Could you check a few things on this model? Use its own coordinates, in mm. Give positions to 0.01 mm unless a question says otherwise; leave off trailing zeros. Order: outer loops, then holes, each group sorted by start corner. A loop starts at its lowest first (then second) coordinate and runs counter-clockwise, first axis right, second up. Notation, with made-up numbers: M 44,-36.5 L 62,-36.5 A26 ccw 62,-11.5 Z; hole C 53.5,-20 d1. An arc over 180 degrees is marked long. Return JSON: item names as keys, results as strings. Group by question number.
```python
from build123d import *

# Parameters (mm, degrees)
SKETCH1_R           = 4
BOSS_EXTRUDE1_DEPTH = 5
CUT_EXTRUDE1_DEPTH  = 114.247516529
SKETCH3_W           = 26
SKETCH3_H           = 1.063316513
BOSS_EXTRUDE2_DEPTH = 5


with BuildPart() as part:
    # Sketch1 → Boss-Extrude1 (new body)
    with BuildSketch(Plane.XY):
        with BuildLine():
            Line((-80, 0), (-17.5, 0))
            ThreePointArc((-17.5, 0), (0, 17.5), (17.5, 0))
            Line((17.5, 0), (80, 0))
            ThreePointArc((80, 0), (0, 80), (-80, 0))
        make_face()
        with Locations((24.874423104, 60.052169613)):
            Circle(SKETCH1_R, mode=Mode.SUBTRACT)
        with Locations((60.052169613, 24.874423104)):
            Circle(SKETCH1_R, mode=Mode.SUBTRACT)
        with Locations((-60.052169613, 24.874423104)):
            Circle(SKETCH1_R, mode=Mode.SUBTRACT)
        with Locations(Location((-24.874423104, 60.052169613, 0), (0, 0, 180))):
            Circle(SKETCH1_R, mode=Mode.SUBTRACT)
    extrude(amount=BOSS_EXTRUDE1_DEPTH)

    # Sketch2 → Cut-Extrude1 (cut, through all)
    with BuildSketch(Plane.XY):
        with BuildLine():
            Line((-12.374368671, 12.374368671), (-56.568542495, 56.568542495))
            Line((-56.568542495, 56.568542495), (-80, 56.568542495))
            Line((-80, 56.568542495), (-80, 0))
            Line((-80, 0), (-17.5, 0))
            ThreePointArc((-17.5, 0), (-16.167891819, 6.696960066), (-12.374368671, 12.374368671))
        make_face()
        with BuildLine():
            Line((80, 0), (80, 56.568542495))
            Line((80, 56.568542495), (56.568542495, 56.568542495))
            Line((56.568542495, 56.568542495), (12.374368671, 12.374368671))
            ThreePointArc((12.374368671, 12.374368671), (16.167891819, 6.696960066), (17.5, 0))
            Line((17.5, 0), (80, 0))
        make_face()
    extrude(amount=CUT_EXTRUDE1_DEPTH, mode=Mode.SUBTRACT)

    # Sketch3 → Boss-Extrude2 (add)
    with BuildSketch(Plane.XY):
        with Locations((0, 79.468341744)):
            Rectangle(SKETCH3_W, SKETCH3_H)
    extrude(amount=BOSS_EXTRUDE2_DEPTH)


solid = part.part
```
1. For pin 1 (1.5 mm diameter, centred on y = 40.5, z = 3.5, fed in from +X); pin 2 (6.5 mm diameter, centred on x = 24.87, y = 60.05, fed in from +Z); pin 3 (0.5 mm diameter, centred on y = 79.5, z = 2.5, fed in from -X), each with a flat end and sliding along its axis, tell me the tip position at first contact or that it passes through.
2. Imagine slicing it at B-B, the plane z = 2.45. Please give me the cut outline in (x, y).
3. I need wall thicknesses on L1, parallel to X at y = 59.5, z = 3.9; L2, parallel to X at y = 60, z = 3; L3, parallel to Y at x = -27, z = 2.2. Which ranges of each line are inside material? Lowest first, please. Write a range as from..to.
4. Imagine slicing it at C-C, the plane y = 43. Please give me the cut outline in (x, z).
5. If we mould it in two halves opening along X, with no side actions, what happens to faces 1 (the flat face through (-1, 47, 0)), 2 (the flat face through (35, 35, 2)), 3 (the cylindrical face through (-24.007, 63.957, 2.465))? For each: pulls with the +X half, pulls with the -X half, needs draft (parallel to the pull), parting line crosses it, or undercut.
6. Imagine slicing it at D-D, the plane x = -43.5. Please give me the cut outline in (y, z).
7. Imagine slicing it at A-A, the plane x = 27. Please give me the cut outline in (y, z), plus the area to 3 significant figures.
Values:
{
 "1": {"pin 1": "stops at x = 41.25", "pin 2": "passes through", "pin 3": "stops at x = -13"},
 "2": {"outline": "M -56.57,56.57 L -12.37,12.37 A17.5 cw 12.37,12.37 L 56.57,56.57 A80 ccw 13,78.94 L 13,80 L -13,80 L -13,78.94 A80 ccw Z; hole C -24.87,60.05 d8; hole C 24.87,60.05 d8"},
 "3": {"L1": "x = -53.48..-28.84, -20.91..20.91, 28.84..53.48", "L2": "x = -52.92..-28.87, -20.87..20.87, 28.87..52.92", "L3": "y = 27..56.66, 63.44..75.31"},
 "4": {"outline": "M -43,0 L 43,0 L 43,5 L -43,5 Z"},
 "5": {"face 1": "needs draft", "face 2": "pulls with the +X half", "face 3": "undercut"},
 "6": {"outline": "M 43.5,0 L 67.14,0 L 67.14,5 L 43.5,5 Z"},
 "7": {"outline": "M 27,0 L 56.66,0 L 56.66,5 L 27,5 Z; M 63.44,0 L 75.31,0 L 75.31,5 L 63.44,5 Z", "area": "208 mm²"}
}
